Geometry: final body of the model. Coordinates: model frame, mm. Face numbers are marked on the shaded views. Give positions to 0.01 mm unless a question says otherwise; leave off trailing zeros. Write each loop counter-clockwise with the first axis right and the second up, starting at its lowest first coordinate (ties: lowest second). Pieces come first, ordered by that corner, then holes. Notation, with made-up numbers: M 60,77 L 114,77 A15 cw 114,104 Z; hole C -16.75,36 d7. An arc over 180 degrees is marked long. One line per question, with ' | ' between items.
from build123d import *

# Parameters (mm, degrees)
SKETCH1_R           = 40
SKETCH1_R_2         = 25
BOSS_EXTRUDE1_DEPTH = 6
SKETCH2_R           = 2.25
CUT_EXTRUDE1_DEPTH  = 57.885850613
CIRPATTERN1_COUNT   = 6


with BuildPart() as part:
    # Sketch1 → Boss-Extrude1 (new body)
    with BuildSketch(Plane.XY):
        Circle(SKETCH1_R)
        Circle(SKETCH1_R_2, mode=Mode.SUBTRACT)
    extrude(amount=BOSS_EXTRUDE1_DEPTH)

    # Sketch2 → Cut-Extrude1 (cut, through all)
    with BuildSketch(Plane.XY):
        with Locations((0, 32.5)):
            Circle(SKETCH2_R)
    cut_extrude1 = extrude(amount=CUT_EXTRUDE1_DEPTH, mode=Mode.SUBTRACT)

    # CirPattern1: Cut-Extrude1 ×6 about axis
    cirpattern1_axis = Axis((0, 0, 6), (0, 0, 1))
    for i in range(1, CIRPATTERN1_COUNT):
        add(cut_extrude1.rotate(cirpattern1_axis, i * 360 / CIRPATTERN1_COUNT), mode=Mode.SUBTRACT)


solid = part.part
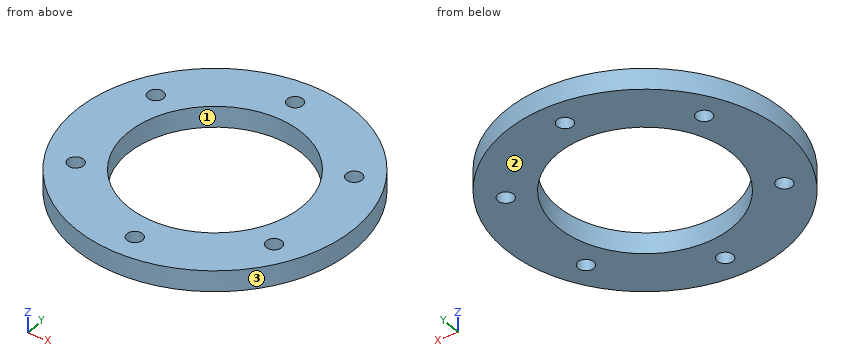
(1) Cut plane A-A, the plane y = 0. Return loops of the section in (x, z).
Working result:
outline: M -40,0 L -25,0 L -25,6 L -40,6 Z; M 25,0 L 40,0 L 40,6 L 25,6 Z
(2) Cut plane B-B, the plane x = 0. Return loops of the section in (y, z).
Working result:
outline: M -40,0 L -34.75,0 L -34.75,6 L -40,6 Z; M -30.25,0 L -25,0 L -25,6 L -30.25,6 Z; M 25,0 L 30.25,0 L 30.25,6 L 25,6 Z; M 34.75,0 L 40,0 L 40,6 L 34.75,6 Z
(3) Material intervals for L1, parallel to Y at x = 0, z = 3.3; L2, parallel to Y at x = -27.5, z = 0.95; L3, parallel to Y at x = 2, z = 2.6, sorted ascending. Write a range as [from, to].
Working result:
L1: y = [-40, -34.75], [-30.25, -25], [25, 30.25], [34.75, 40] | L2: y = [-29.05, -18.41], [-14.09, 14.09], [18.41, 29.05] | L3: y = [-39.95, -33.53], [-31.47, -24.92], [24.92, 31.47], [33.53, 39.95]
(4) Draft query along Y for the marked faces 1, 2 and 3. Return one class per face: released by +Y, released by -Y, zero draft, split by the parting line, or undercut.
Working result:
face 1: undercut | face 2: zero draft | face 3: split by the parting line
(5) Cut plane D-D, the plane x = -22.5. Return loops of the section in (y, z).
Working result:
outline: M -33.07,0 L -10.9,0 L -10.9,6 L -33.07,6 Z; M 10.9,0 L 33.07,0 L 33.07,6 L 10.9,6 Z
(6) Cut plane C-C, the plane z = 4.1. Return loops of the section in (x, y), then the cut area to 3 significant figures.
Working result:
outline: C 0,0 d80; hole C -28.15,-16.25 d4.5; hole C -28.15,16.25 d4.5; hole C 0,0 d50; hole C 0,-32.5 d4.5; hole C 0,32.5 d4.5; hole C 28.15,-16.25 d4.5; hole C 28.15,16.25 d4.5 | area: 2,970 mm^2
(7) First-contact query: P1, Ø2, axis at x = -4, z = 2, coming from the +Y side. Flat tip, straight axial feed; report the tip coordinate or a pass-through.
Working result:
P1: stops at y = 39.89
